Geometry check sheet. Reference: drawing and pictorial views, mm from the part's lowest x, y, z. Round coordinates to 2 decimals unless told otherwise and drop trailing zeros. Order: outer loops, then holes, each group sorted by start corner. A loop starts at its lowest first (then second) coordinate and runs counter-clockwise, first axis right, second up.
(1) Cross-section at A-A on x = 17.5. Count the separate pieces of the cut face and the enclosed holes in it.
(2) Cross-section at B-B on z = 0.95. Enter the section's corners in (x, y).
(3) Gauge pin test, flat end, axial feed: P1, Ø2.5, axis at x = 16.48, y = 20.4, coming from the -Z side. Record the tip position at first contact, or that the pin passes through.
(4) Thickness scan on L1, parallel to X at y = 20.5, z = 0.6 (1 decimal); L2, parallel to Y at x = 16.5, z = 1.15 (1 decimal); L3, parallel to X at y = 21.75, z = 1.6 (1 decimal). Record the ranges inside material, lowest first.
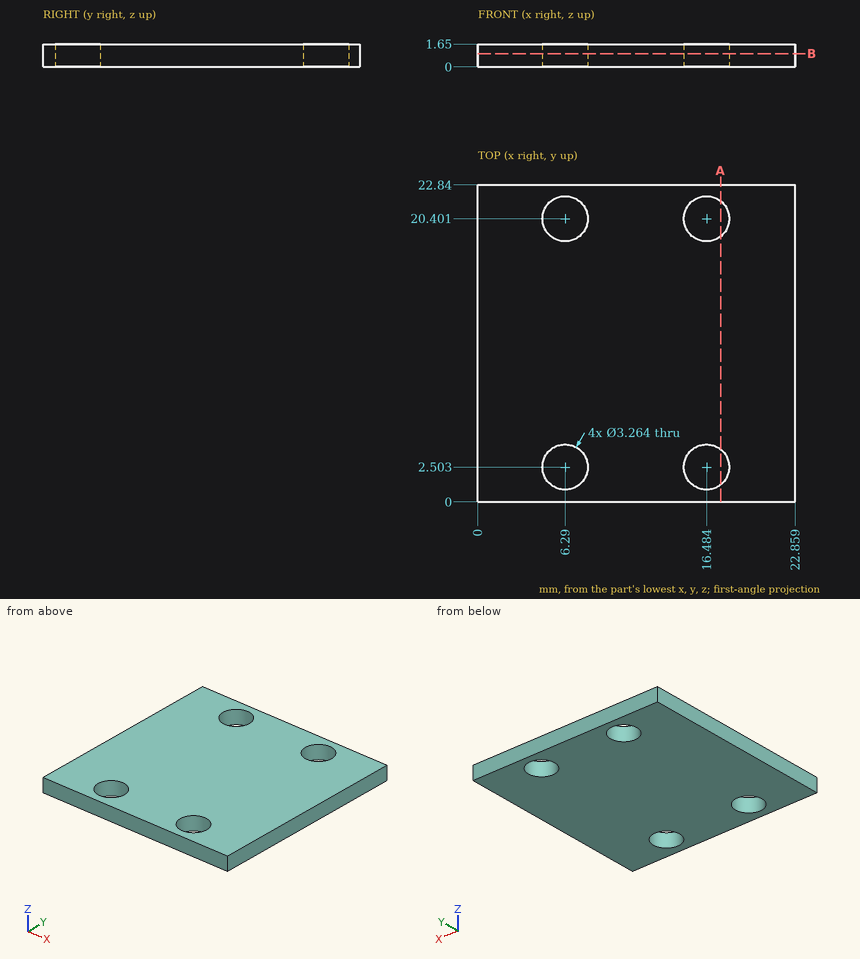
Found:
1. separate pieces: 3
1. enclosed holes: 0
2. outline: (0, 0) - (22.86, 0) - (22.86, 22.84) - (0, 22.84) - close; hole circle Ø3.26 at (6.29, 2.5); hole circle Ø3.26 at (6.29, 20.4); hole circle Ø3.26 at (16.48, 2.5); hole circle Ø3.26 at (16.48, 20.4)
3. P1: passes through
4. L1: x = 0 to 4.7, 7.9 to 14.9, 18.1 to 22.9
4. L2: y = 0 to 0.9, 4.1 to 18.8, 22 to 22.8
4. L3: x = 0 to 5.4, 7.2 to 15.6, 17.4 to 22.9
